Can you work these out from the drawing? Everything is in mm from the part's minimum corner. Round coordinates to 2 decimals unless told otherwise and drop trailing zeros. Loops run counter-clockwise (first coordinate to the right, second up) from the corner with the lowest first, then second, coordinate; pieces in that order, holes last. Notation, with made-up numbers: (74.5, 80.25) -> (104.5, 80.25) arc R24 ccw to (104.5, 105.25) -> close; hole circle Ø10 at (-20.75, 61). An arc over 180 degrees is marked (long way). Use CSV: the item, a comma, the result in double quotes. Start each with the question number.
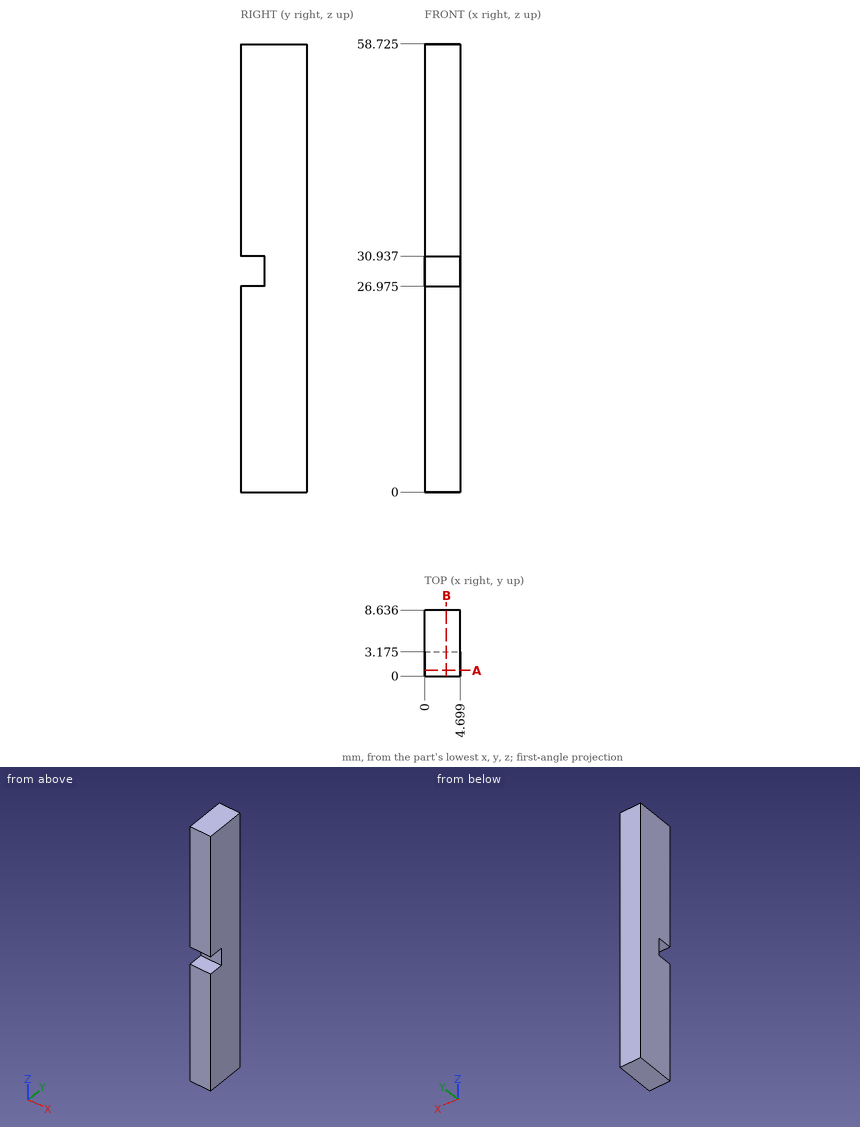
1. Suppose I cut it at B-B (x = 2.85). List the corners of the cut face in (y, z) for me (1 decimal), then the cut area to 3 significant figures.
2. Suppose I cut it at A-A (y = 0.75). List the corners of the cut face in (x, z) for me (1 decimal).
3. If I drill on L1, parallel to Z at x = 2.3, y = 1.75 (1 decimal); L2, parallel to Y at x = 1.55, z = 28 (3 decimals), over which ranges is the centre line in solid material (lowest first)?
Geometry check:
1,outline,"(0, 0) -> (8.6, 0) -> (8.6, 58.7) -> (0, 58.7) -> (0, 30.9) -> (3.2, 30.9) -> (3.2, 27) -> (0, 27) -> close"
1,area,"495 mm²"
2,outline,"(0, 0) -> (4.7, 0) -> (4.7, 27) -> (0, 27) -> close; (0, 30.9) -> (4.7, 30.9) -> (4.7, 58.7) -> (0, 58.7) -> close"
3,L1,"z = 0 to 27, 30.9 to 58.7"
3,L2,"y = 3.175 to 8.636"
